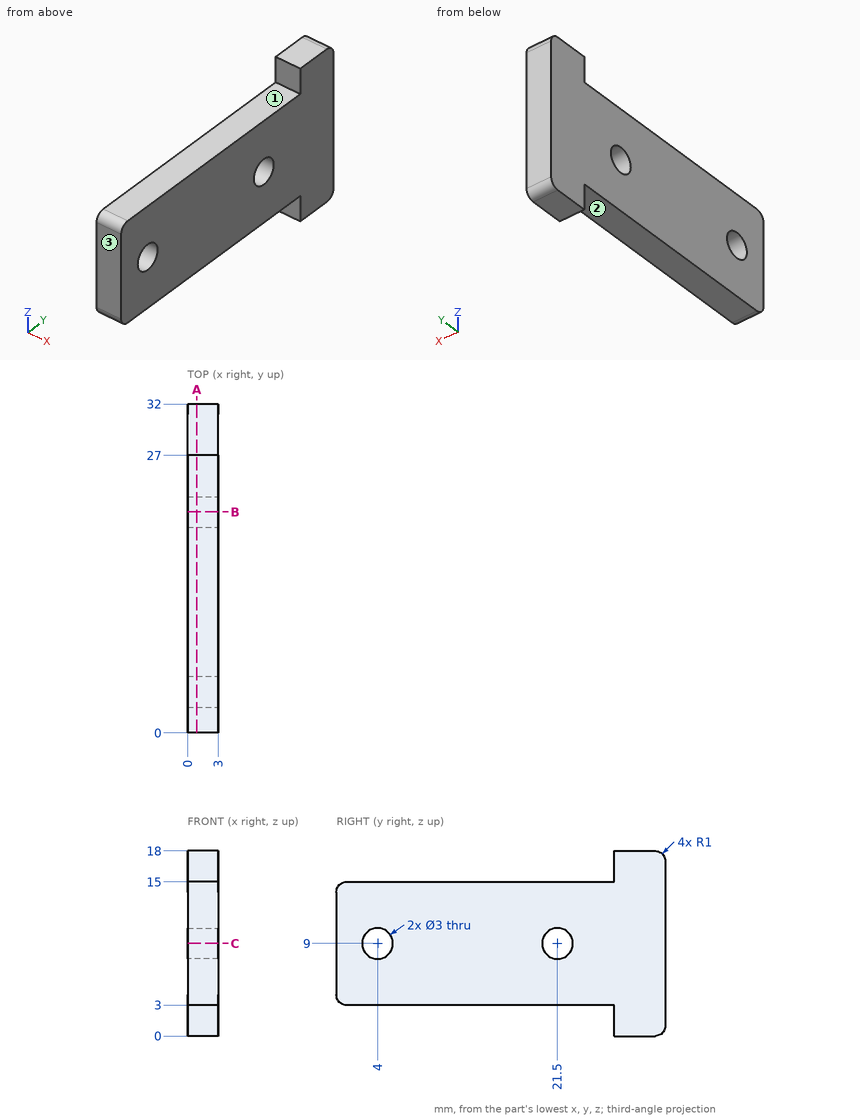
Input: dimensioned drawing with shaded views. Units: mm. Origin: part minimum x, y, z. A direction names the side the tool comes from. Round coordinates to 2 decimals unless told otherwise and drop trailing zeros. Loops run counter-clockwise (first coordinate to the right, second up) from the corner with the lowest first, then second, coordinate; pieces in that order, holes last. Notation, with made-up numbers: (-19, 4) -> (12, 4) arc R37 cw to (12, 40) -> close; hole circle Ø11 at (5, -27.75). An arc over 180 degrees is marked (long way). Answer as a JSON object with one key per item and string values. Group by question number.
Q1. Ray query, line 1 (Y direction, x = 1.2, z = 9); line 2 (Y direction, x = 1.2, z = 15.75); line 3 (Z direction, x = 1.4, y = 6). Return the intervals inside material, ascending. Write a range as from..to.
Q2. Section query A-A (x = 0.9). Output: boundary loops of the cut face in (y, z), plus the area to 3 significant figures.
Q3. Contact query for flat-ended pins moving along their axis: P1, Ø1, axis at x = 1.5, y = 17.5, coming from the -Z side; P2, Ø1.5, axis at x = 2, z = 16.5, coming from the -Y side; P3, Ø1.5, axis at x = 1.5, y = 19.5, coming from the +Z side. Output: stop coordinate, or through.
Q4. Access query for the marked faces 1, 2 and 3. Directions: +Z, -Z, +X, -X, +Y, -Y. A direction counts if a zero-diameter tool reaches every point of the face in a straight line with its end or side. Return the directions, or none.
Q5. Section query B-B (y = 21.5). Output: boundary loops of the cut face in (x, z), plus the area to 3 significant figures.
Q6. Section query C-C (z = 9). Output: boundary loops of the cut face in (x, y), plus the area to 3 significant figures.
Completed:
{
 "1": {"line 1": "0..2.5, 5.5..20, 23..32", "line 2": "27..32", "line 3": "3..15"},
 "2": {"outline": "(0, 4) arc R1 ccw to (1, 3) -> (27, 3) -> (27, 0) -> (31, 0) arc R1 ccw to (32, 1) -> (32, 17) arc R1 ccw to (31, 18) -> (27, 18) -> (27, 15) -> (1, 15) arc R1 ccw to (0, 14) -> close; hole circle Ø3 at (4, 9); hole circle Ø3 at (21.5, 9)", "area": "399 mm²"},
 "3": {"P1": "z = 3", "P2": "y = 27", "P3": "z = 15"},
 "4": {"face 1": "+Z, +X, -X, -Y", "face 2": "-Z, +X, -X, -Y", "face 3": "+Z, -Z, +X, -X, -Y"},
 "5": {"outline": "(0, 3) -> (3, 3) -> (3, 7.5) -> (0, 7.5) -> close; (0, 10.5) -> (3, 10.5) -> (3, 15) -> (0, 15) -> close", "area": "27.0 mm²"},
 "6": {"outline": "(0, 0) -> (3, 0) -> (3, 2.5) -> (0, 2.5) -> close; (0, 5.5) -> (3, 5.5) -> (3, 20) -> (0, 20) -> close; (0, 23) -> (3, 23) -> (3, 32) -> (0, 32) -> close", "area": "78.0 mm²"}
}
